The figure shows three views and two pictorial views of one solid part (mm, origin at its lowest corner). Answer the questions. A direction names the side the tool comes from. Round coordinates to 2 decimals unless told otherwise and drop trailing zeros. Write each loop counter-clockwise with the first axis right and the second up, starting at its lowest first coordinate (ties: lowest second). Pieces come first, ordered by that corner, then holes. Notation, with made-up numbers: M 25.25,-15 L 39.25,-15 A23 cw 39.25,2 Z; hole C 16,76.5 d4. An arc over 180 degrees is marked long. Answer in a Markdown table with one row per item.
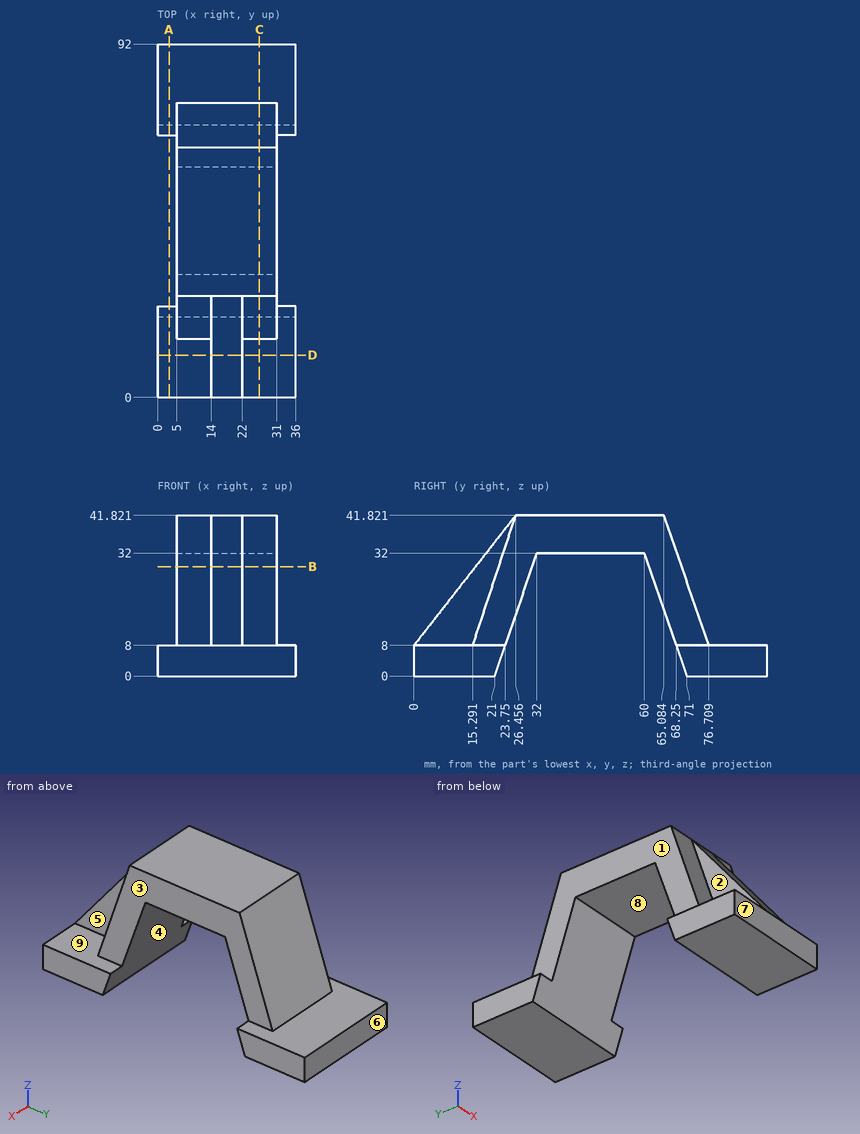
1. A tool of negligible diameter and unlimited length cuts with its end or side. For the marked faces 1, 2, 3, 4 and 5, from which of +Z, -Z, +X, -X, +Y, -Y can it reach the whole face along a straight path? Write none if from no direction.
Calculated:
| item | result |
|---|---|
| face 1 | +Z, -X, +Y, -Y |
| face 2 | +Z, -X, -Y |
| face 3 | +Z, +X, +Y, -Y |
| face 4 | -Z, +X, -X |
| face 5 | +Z, +X, -Y |
2. The part is cut by section C-C (x = 26.5). Determine the outline of the cut face in (y, z).
Calculated:
| item | result |
|---|---|
| outline | M 0,0 L 21,0 L 32,32 L 60,32 L 71,0 L 92,0 L 92,8 L 76.71,8 L 65.08,41.82 L 26.46,41.82 L 15.29,8 L 0,8 Z |
3. The part is cut by section B-B (z = 28.5). Determine the outline of the cut face in (x, y).
Calculated:
| item | result |
|---|---|
| outline | M 5,22.06 L 14,22.06 L 14,16.04 L 22,16.04 L 22,22.06 L 31,22.06 L 31,30.8 L 5,30.8 Z; M 5,61.2 L 31,61.2 L 31,69.66 L 5,69.66 Z |
4. The part is cut by section A-A (x = 3). Determine the outline of the cut face in (y, z).
Calculated:
| item | result |
|---|---|
| outline | M 0,0 L 21,0 L 23.75,8 L 0,8 Z; M 68.25,8 L 71,0 L 92,0 L 92,8 Z |
5. Given pin 1 (21 mm diameter, centred on y = 13, z = 29, fed in from +X); pin 2 (21 mm diameter, centred on y = 10.5, z = 23.5, fed in from -X), each flat-ended and moving along its own axis, determine where each tip first touches the part or whether it passes through.
Calculated:
| item | result |
|---|---|
| pin 1 | stops at x = 31 |
| pin 2 | stops at x = 5 |
6. Determine the mould class of the marked faces 6, 7, 8 and 9 for opening direction Y: released by +Y, released by -Y, zero draft, split by the parting line, or undercut.
Calculated:
| item | result |
|---|---|
| face 6 | released by +Y |
| face 7 | released by -Y |
| face 8 | undercut |
| face 9 | zero draft |
7. Consider line 1 along Z through (x, y) = (30.5, 5); line 2 along X through (y, z) = (14, 14.5); line 3 along Y through (x, z) = (20.5, 22.5) (1 decimal). Determine where each line is inside the solid, lowest interval first. Write a range as from..to.
Calculated:
| item | result |
|---|---|
| line 1 | z = 0..8 |
| line 2 | x = 14..22 |
| line 3 | y = 11.3..28.7, 63.3..71.7 |
8. The part is cut by section D-D (y = 11). Determine the outline of the cut face in (x, z).
Calculated:
| item | result |
|---|---|
| outline | M 0,0 L 36,0 L 36,8 L 22,8 L 22,22.06 L 14,22.06 L 14,8 L 0,8 Z |
